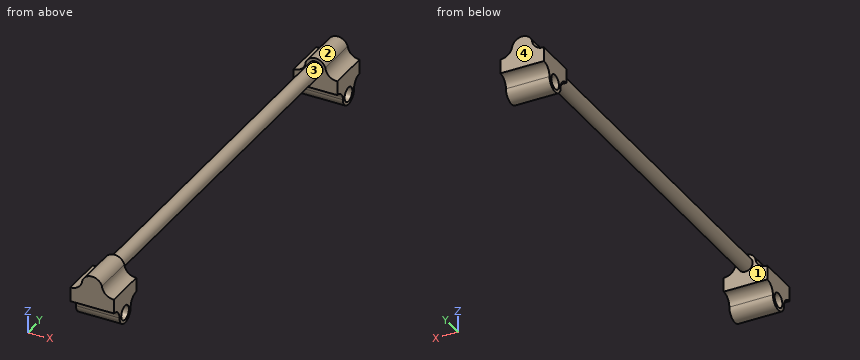
```python
from build123d import *

# Parameters (mm, degrees)
SKETCH011_R  = 6.9
PAD001_DEPTH = 42
SKETCH012_R  = 6.9
PAD002_DEPTH = 42
SKETCH014_R  = 6.9
PAD004_DEPTH = 20
SKETCH015_R  = 6.9
PAD005_DEPTH = 20
SKETCH016_R  = 6.9
PAD006_DEPTH = 440


with BuildPart() as x_axis_sled1:
    # Sketch011 → Pad001 (new body)
    with BuildSketch(Plane.YZ):
        with BuildLine():
            Line((-20, 16.9), (20, 16.9))
            Line((20, 16.9), (20, 10))
            ThreePointArc((20, 10), (12.928932, 7.071068), (10, 0))
            ThreePointArc((-10, 0), (0, -9.999999), (10, 0))
            ThreePointArc((-10, 0), (-12.928932, 7.071068), (-20, 10))
            Line((-20, 10), (-20, 16.9))
        make_face()
        Circle(SKETCH011_R, mode=Mode.SUBTRACT)
    extrude(amount=PAD001_DEPTH)


with BuildPart() as x_axis_sled2:
    # Sketch012 → Pad002 (new body)
    with BuildSketch(Plane(origin=(0, 400, 0), x_dir=(0, 1, 0), z_dir=(1, 0, 0))):
        with BuildLine():
            Line((-20, 16.9), (20, 16.9))
            Line((20, 16.9), (20, 10))
            ThreePointArc((20, 10), (12.928932, 7.071068), (10, 0))
            ThreePointArc((-10, 0), (0, -9.999999), (10, 0))
            ThreePointArc((-10, 0), (-12.928932, 7.071068), (-20, 10))
            Line((-20, 10), (-20, 16.9))
        make_face()
        Circle(SKETCH012_R, mode=Mode.SUBTRACT)
    extrude(amount=PAD002_DEPTH)


with BuildPart() as y_axis_socket1:
    # Sketch014 → Pad004 (new body, symmetric)
    with BuildSketch(Plane.XZ):
        with BuildLine():
            Line((0, 23.8), (0, 16.9))
            Line((0, 16.9), (42, 16.9))
            Line((42, 16.9), (42, 23.8))
            ThreePointArc((30.507366, 33.8), (34.242407, 26.488514), (42, 23.8))
            ThreePointArc((30.507366, 33.8), (21, 40.7), (11.492634, 33.8))
            ThreePointArc((0, 23.8), (7.757593, 26.488514), (11.492634, 33.8))
        make_face()
        with Locations((21, 30.7)):
            Circle(SKETCH014_R, mode=Mode.SUBTRACT)
    extrude(amount=PAD004_DEPTH, both=True)


with BuildPart() as y_axis_socket2:
    # Sketch015 → Pad005 (new body, symmetric)
    with BuildSketch(Plane.XZ.offset(-400)):
        with BuildLine():
            Line((0, 23.8), (0, 16.9))
            Line((0, 16.9), (42, 16.9))
            Line((42, 16.9), (42, 23.8))
            ThreePointArc((30.507366, 33.8), (34.242407, 26.488514), (42, 23.8))
            ThreePointArc((30.507366, 33.8), (21, 40.7), (11.492634, 33.8))
            ThreePointArc((0, 23.8), (7.757593, 26.488514), (11.492634, 33.8))
        make_face()
        with Locations((21, 30.7)):
            Circle(SKETCH015_R, mode=Mode.SUBTRACT)
    extrude(amount=PAD005_DEPTH, both=True)


with BuildPart() as y_rail:
    # Sketch016 → Pad006 (new body)
    with BuildSketch(Plane.XZ.offset(20)):
        with Locations((21, 30.7)):
            Circle(SKETCH016_R)
    extrude(amount=-PAD006_DEPTH)

    # Fusion: union X_Axis_Sled1, X_Axis_Sled2, Y_Axis_Socket1, Y_Axis_Socket2
    add(x_axis_sled1.part)
    add(x_axis_sled2.part)
    add(y_axis_socket1.part)
    add(y_axis_socket2.part)


solid = y_rail.part
```
Work out the finished part from the listing and answer in its coordinate system (mm). Face numbers are marked on the shaded views. Coordinates: 2 decimals unless noted, no trailing zeros. Write each loop counter-clockwise with the first axis right and the second up, starting at its lowest first coordinate (ties: lowest second). Pieces come first, ordered by that corner, then holes. Notation, with made-up numbers: (49, -14) - (63, -14) arc R16 ccw to (63, 15) - close; hole circle Ø4 at (16.25, 43.5). An arc over 180 degrees is marked (long way). Answer as a JSON object with one key per item and string values.
Q1. Given pin 1 Ø2 at (y, z) = (77.5, 28.5) entering from +X; pin 2 Ø16 at (y, z) = (0, 0) entering from -X; pin 3 Ø6 at (x, z) = (11, 4) entering from -Y, each flat-ended and moving along its own axis, determine where each tip first touches the part or whether it passes through.
Results list:
{"pin 1": "stops at x = 27.79", "pin 2": "stops at x = 0", "pin 3": "stops at y = -12.86"}
Q2. Find section C-C (z = 14). Write down the section's boundary in (x, y).
Results list:
{"outline": "(0, -20) - (42, -20) - (42, 20) - (0, 20) - close; (0, 380) - (42, 380) - (42, 420) - (0, 420) - close"}
Q3. For a pull along Y with two mould halves and no side action, classify the marked faces 1, 2, 3 and 4 as pulls with the +Y half, pulls with the -Y half, needs draft (parallel to the pull), parting line crosses it, or undercut.
Results list:
{"face 1": "undercut", "face 2": "needs draft", "face 3": "undercut", "face 4": "pulls with the +Y half"}
Q4. Find section A-A (y = 400). Write down the section's boundary in (x, z), plus the area to 3 significant figures.
Results list:
{"outline": "(0, -10) - (42, -10) - (42, -6.9) - (0, -6.9) - close; (0, 6.9) - (42, 6.9) - (42, 23.8) arc R11 cw to (30.51, 33.8) arc R10 ccw to (11.49, 33.8) arc R11 cw to (0, 23.8) - close", "area": "1,180 mm^2"}
Q5. Consider L1, parallel to Y at x = 10, z = 19; L2, parallel to Y at x = 32, z = 5.5; L3, parallel to Y at x = 25, z = -6. Determine where each line is inside the solid, lowest interval first. Write a range as from..to.
Results list:
{"L1": "y = -20..20, 380..420", "L2": "y = -11.65..-4.17, 4.17..11.65, 388.35..395.83, 404.17..411.65", "L3": "y = -8..-3.41, 3.41..8, 392..396.59, 403.41..408"}
Q6. Find section B-B (x = 38). Write down the section's boundary in (y, z).
Results list:
{"outline": "(-20, 10) arc R10 cw to (-10, 0) arc R10 ccw to (10, 0) arc R10 cw to (20, 10) - (20, 24.35) - (-20, 24.35) - close; (380, 10) arc R10 cw to (390, 0) arc R10 ccw to (410, 0) arc R10 cw to (420, 10) - (420, 24.35) - (380, 24.35) - close; hole circle Ø13.8 at (0, 0); hole circle Ø13.8 at (400, 0)"}
Q7. Find section D-D (x = 21). Write down the section's boundary in (y, z).
Results list:
{"outline": "(-20, 10) arc R10 cw to (-10, 0) arc R10 ccw to (10, 0) arc R10 cw to (20, 10) - (20, 23.8) - (380, 23.8) - (380, 10) arc R10 cw to (390, 0) arc R10 ccw to (410, 0) arc R10 cw to (420, 10) - (420, 40.7) - (380, 40.7) - (380, 37.6) - (20, 37.6) - (20, 40.7) - (-20, 40.7) - close; hole circle Ø13.8 at (0, 0); hole circle Ø13.8 at (400, 0)"}
